Source: CAD feature listing. Evaluate the final solid. Frame: model axes, mm. Face numbers are marked on the shaded views. A direction names the side the tool comes from. Give positions to 0.01 mm unless a question says otherwise; leave off trailing zeros. Order: outer loops, then holes, each group sorted by start corner. A loop starts at its lowest first (then second) coordinate and runs counter-clockwise, first axis right, second up. Notation, with made-up numbers: (-8.75, 53) -> (5.25, 53) arc R16 cw to (5.25, 58) -> close; hole circle Ø6 at (8, -22). An arc over 180 degrees is marked (long way). Answer in a Markdown table with one row per item.
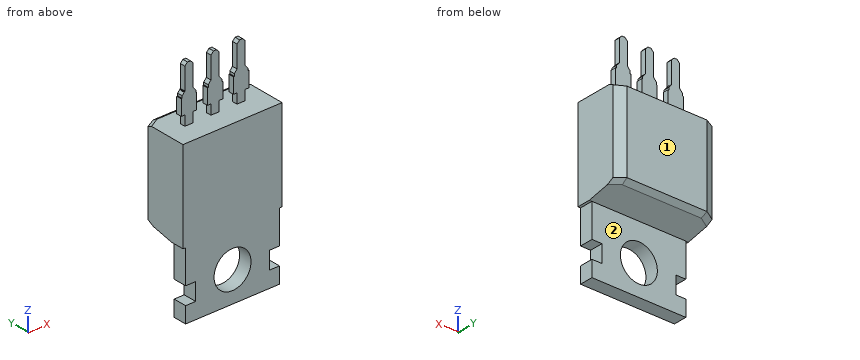
```python
from build123d import *
from OCP.BRepFilletAPI import BRepFilletAPI_MakeChamfer

# Parameters (mm, degrees)
EXTRUDE1_DEPTH      = 4.826
EXTRUDE1_DEPTH_BACK = 4.826
SKETCH10_R          = 1.8
SKETCH10_W          = 1.233836604
SKETCH10_H          = 1.6931216
EXTRUDE5_DEPTH      = 16.428369203
SKETCH6_W           = 0.8
SKETCH6_H           = 0.52
EXTRUDE6_DEPTH      = 5.38
EXTRUDE7_START      = -0.52
EXTRUDE7_DEPTH      = 0.52
CHAMFER1_SIZE       = 0.254
SKETCH12_W          = 7.379682426
SKETCH12_H          = 2.736118788
EXTRUDE8_DEPTH      = 0.254
SKETCH13_W          = 7.379682426
SKETCH13_H          = 2.736118788
EXTRUDE9_DEPTH      = 0.254
CHAMFER2_SIZE       = 0.508
CHAMFER2_SIZE2      = 0.91645626
CHAMFER3_SIZE       = 0.2032
CHAMFER3_SIZE2      = 0.366582504
CHAMFER3_SIZE2_2    = 0.605677555
CHAMFER3_SIZE2_3    = 0.557834937
EXTRUDE10_DEPTH     = 1.016


with BuildPart() as part:
    # Sketch2 → Extrude1 (new, two sides: drawn at the far end of the back side and taken through both)
    with BuildSketch(Plane(origin=(0, 0, 0), x_dir=(0, 0, -1), z_dir=(1, 0, 0)).offset(-EXTRUDE1_DEPTH_BACK)):
        Polygon((14.3005, 0), (-1.0795, 0), (-1.0795, 4.5), (7.124012877, 4.5), (7.8005, 1.3), (14.3005, 1.3), align=None)
    extrude(amount=EXTRUDE1_DEPTH + EXTRUDE1_DEPTH_BACK)

    # Sketch10 → Extrude5 (cut, through all)
    with BuildSketch(Plane(origin=(0, 1.3, 0), x_dir=(1, 0, 0), z_dir=(0, 1, 0))):
        with Locations(Location((0, 11.3505, 0), (0, 0, 270))):
            Circle(SKETCH10_R)
        with Locations((-4.209081698, 11.892729701)):
            Rectangle(SKETCH10_W, SKETCH10_H)
        with Locations((4.209081698, 11.892729701)):
            Rectangle(SKETCH10_W, SKETCH10_H)
    extrude(amount=-EXTRUDE5_DEPTH, mode=Mode.SUBTRACT)

    # Sketch6 → Extrude6 (add)
    with BuildSketch(Plane.XY.offset(1.0795)):
        with Locations((2.54, 2.25)):
            Rectangle(SKETCH6_W, SKETCH6_H)
        with Locations((-2.54, 2.25)):
            Rectangle(SKETCH6_W, SKETCH6_H)
        with Locations((0, 2.25)):
            Rectangle(SKETCH6_W, SKETCH6_H)
    extrude(amount=EXTRUDE6_DEPTH)

    # Sketch11 → Extrude7 (add)
    with BuildSketch(Plane(origin=(0, 2.51, 0), x_dir=(1, 0, 0), z_dir=(0, 1, 0)).offset(EXTRUDE7_START)):
        Polygon((-2.94, -2.0475), (-3.29, -2.0475), (-3.29, -3.5395), (-3.2004, -3.5395), (-3.2004, -3.7747), (-2.94, -4.0795), align=None)
        Polygon((-1.79, -2.0475), (-2.14, -2.0475), (-2.14, -4.0795), (-1.8796, -3.7747), (-1.8796, -3.5395), (-1.79, -3.5395), align=None)
        Polygon((-0.4, -2.0475), (-0.75, -2.0475), (-0.75, -3.5395), (-0.6604, -3.5395), (-0.6604, -3.7747), (-0.4, -4.0795), align=None)
        Polygon((0.75, -2.0475), (0.4, -2.0475), (0.4, -4.0795), (0.6604, -3.7747), (0.6604, -3.5395), (0.75, -3.5395), align=None)
        Polygon((2.14, -2.0475), (1.79, -2.0475), (1.79, -3.5395), (1.8796, -3.5395), (1.8796, -3.7747), (2.14, -4.0795), align=None)
        Polygon((3.29, -2.0475), (2.94, -2.0475), (2.94, -4.0795), (3.2004, -3.7747), (3.2004, -3.5395), (3.29, -3.5395), align=None)
    extrude(amount=EXTRUDE7_DEPTH)

    # Chamfer1
    chamfer1_edges = [part.edges().sort_by_distance(p)[0] for p in [
        (-2.14, 2.25, 6.4595),
        (-2.94, 2.25, 6.4595),
        (2.94, 2.25, 6.4595),
        (2.14, 2.25, 6.4595),
        (0.4, 2.25, 6.4595),
        (-0.4, 2.25, 6.4595),
    ]]
    chamfer(chamfer1_edges, length=CHAMFER1_SIZE)

    # Sketch12 → Extrude8 (cut)
    with BuildSketch(Plane.ZY.offset(4.826)):
        with Locations((-11.490341213, 1.368059394)):
            Rectangle(SKETCH12_W, SKETCH12_H)
    extrude(amount=-EXTRUDE8_DEPTH, mode=Mode.SUBTRACT)

    # Sketch13 → Extrude9 (cut)
    with BuildSketch(Plane(origin=(4.826, 0, 0), x_dir=(0, 0, -1), z_dir=(1, 0, 0))):
        with Locations((11.490341213, 1.368059394)):
            Rectangle(SKETCH13_W, SKETCH13_H)
    extrude(amount=-EXTRUDE9_DEPTH, mode=Mode.SUBTRACT)

    # Chamfer2: one chamfer whose edges measure the first distance from different faces: ONE call of the kernel's chamfer builder (chamfer() names one face for all edges)
    chamfer2_edges_1 = [part.edges().sort_by_distance(p)[0] for p in [
        (-4.826, 4.5, -3.022256439),
    ]]
    chamfer2_side_1 = [part.faces().sort_by_distance(p)[0] for p in [
        (-4.826, 2.217055195, -3.243165334),
    ]]
    chamfer2_edges_2 = [part.edges().sort_by_distance(p)[0] for p in [
        (4.826, 4.5, -3.022256439),
    ]]
    chamfer2_side_2 = [part.faces().sort_by_distance(p)[0] for p in [
        (4.826, 2.217055195, -3.243165334),
    ]]
    chamfer2 = BRepFilletAPI_MakeChamfer(part.part.solid().wrapped)
    for e in chamfer2_edges_1:
        chamfer2.Add(CHAMFER2_SIZE, CHAMFER2_SIZE2, e.wrapped, chamfer2_side_1[0].wrapped)  # the first distance lies on this face
    for e in chamfer2_edges_2:
        chamfer2.Add(CHAMFER2_SIZE, CHAMFER2_SIZE2, e.wrapped, chamfer2_side_2[0].wrapped)  # the first distance lies on this face
    add(Compound.cast(chamfer2.Shape()), mode=Mode.REPLACE)

    # Chamfer3: one chamfer whose edges measure the first distance from different faces: ONE call of the kernel's chamfer builder (chamfer() names one face for all edges)
    chamfer3_edges_1 = [part.edges().sort_by_distance(p)[0] for p in [
        (0, 4.5, 1.0795),
    ]]
    chamfer3_side_1 = [part.faces().sort_by_distance(p)[0] for p in [
        (0, 4.5, -3.022256439),
    ]]
    chamfer3_edges_2 = [part.edges().sort_by_distance(p)[0] for p in [
        (-4.36777187, 4.246, 1.0795),
    ]]
    chamfer3_side_2 = [part.faces().sort_by_distance(p)[0] for p in [
        (-4.368765147, 4.245449417, -3.049162718),
    ]]
    chamfer3_edges_3 = [part.edges().sort_by_distance(p)[0] for p in [
        (4.36777187, 4.246, 1.0795),
    ]]
    chamfer3_side_3 = [part.faces().sort_by_distance(p)[0] for p in [
        (4.368765147, 4.245449417, -3.049162718),
    ]]
    chamfer3_edges_4 = [part.edges().sort_by_distance(p)[0] for p in [
        (0, 4.5, -7.124012877),
    ]]
    chamfer3_side_4 = [part.faces().sort_by_distance(p)[0] for p in [
        (0, 4.5, -3.022256439),
    ]]
    chamfer3_edges_5 = [part.edges().sort_by_distance(p)[0] for p in [
        (-4.36777187, 4.246, -7.177709043),
    ]]
    chamfer3_side_5 = [part.faces().sort_by_distance(p)[0] for p in [
        (-4.368765147, 4.245449417, -3.049162718),
    ]]
    chamfer3_edges_6 = [part.edges().sort_by_distance(p)[0] for p in [
        (4.36777187, 4.246, -7.177709043),
    ]]
    chamfer3_side_6 = [part.faces().sort_by_distance(p)[0] for p in [
        (4.368765147, 4.245449417, -3.049162718),
    ]]
    chamfer3 = BRepFilletAPI_MakeChamfer(part.part.solid().wrapped)
    for e in chamfer3_edges_1:
        chamfer3.Add(CHAMFER3_SIZE, CHAMFER3_SIZE2, e.wrapped, chamfer3_side_1[0].wrapped)  # the first distance lies on this face
    for e in chamfer3_edges_2:
        chamfer3.Add(CHAMFER3_SIZE, CHAMFER3_SIZE2, e.wrapped, chamfer3_side_2[0].wrapped)  # the first distance lies on this face
    for e in chamfer3_edges_3:
        chamfer3.Add(CHAMFER3_SIZE, CHAMFER3_SIZE2, e.wrapped, chamfer3_side_3[0].wrapped)  # the first distance lies on this face
    for e in chamfer3_edges_4:
        chamfer3.Add(CHAMFER3_SIZE, CHAMFER3_SIZE2_2, e.wrapped, chamfer3_side_4[0].wrapped)  # the first distance lies on this face
    for e in chamfer3_edges_5:
        chamfer3.Add(CHAMFER3_SIZE, CHAMFER3_SIZE2_3, e.wrapped, chamfer3_side_5[0].wrapped)  # the first distance lies on this face
    for e in chamfer3_edges_6:
        chamfer3.Add(CHAMFER3_SIZE, CHAMFER3_SIZE2_3, e.wrapped, chamfer3_side_6[0].wrapped)  # the first distance lies on this face
    add(Compound.cast(chamfer3.Shape()), mode=Mode.REPLACE)

    # Sketch15 → Extrude10 (add)
    with BuildSketch(Plane.XY.offset(4.0795)):
        with BuildLine():
            Line((-2.14, 2.51), (-2.94, 2.51))
            ThreePointArc((-2.94, 2.51), (-3.017074418, 2.25), (-2.94, 1.99))
            Line((-2.94, 1.99), (-2.14, 1.99))
            ThreePointArc((-2.14, 1.99), (-2.062925582, 2.25), (-2.14, 2.51))
        make_face()
    extrude(amount=-EXTRUDE10_DEPTH)


solid = part.part
```
(1) Section query C-C (z = -10.75). Return the cut outline in (x, y), plus the area to 3 significant figures.
A:
| item | result |
|---|---|
| outline | (-4.57, 0) -> (-1.7, 0) -> (-1.7, 1.3) -> (-4.57, 1.3) -> close; (1.7, 0) -> (4.57, 0) -> (4.57, 1.3) -> (1.7, 1.3) -> close |
| area | 7.48 mm^2 |
(2) Section query A-A (z = 2.25). Return the cut outline in (x, y).
A:
| item | result |
|---|---|
| outline | (-3.29, 1.99) -> (-1.79, 1.99) -> (-1.79, 2.51) -> (-3.29, 2.51) -> close; (-0.75, 1.99) -> (0.75, 1.99) -> (0.75, 2.51) -> (-0.75, 2.51) -> close; (1.79, 1.99) -> (3.29, 1.99) -> (3.29, 2.51) -> (1.79, 2.51) -> close |
(3) Ray query, probe 1 along X at (y, z) = (2.05, 5); probe 2 along Y at (x, z) = (-4, -11); probe 3 along Y at (x, z) = (3.25, 3). Return the intervals inside material, ascending.
A:
| item | result |
|---|---|
| probe 1 | x = -2.94 to -2.14, -0.4 to 0.4, 2.14 to 2.94 |
| probe 2 | y = 0 to 1.3 |
| probe 3 | y = 1.99 to 2.51 |
(4) Section query B-B (y = 0.4). Return the cut outline in (x, z), plus the area to 3 significant figures.
A:
| item | result |
|---|---|
| outline | (-4.83, -7.8) -> (-4.57, -7.8) -> (-4.57, -11.05) -> (-3.59, -11.05) -> (-3.59, -12.74) -> (-4.57, -12.74) -> (-4.57, -14.3) -> (4.57, -14.3) -> (4.57, -12.74) -> (3.59, -12.74) -> (3.59, -11.05) -> (4.57, -11.05) -> (4.57, -7.8) -> (4.83, -7.8) -> (4.83, 1.08) -> (-4.83, 1.08) -> close; hole circle Ø3.6 at (0, -11.35) |
| area | 132 mm^2 |
(5) Access query for the marked faces 1 and 2. Directions: +Z, -Z, +X, -X, +Y, -Y. A direction counts if a zero-diameter tool reaches every point of the face in a straight line with its end or side. Return the directions, or none.
A:
| item | result |
|---|---|
| face 1 | +Z, -Z, +X, -X, +Y |
| face 2 | -Z, +X, -X, +Y |
(6) Section query D-D (y = 3.1). Return the cut outline in (x, z).
A:
| item | result |
|---|---|
| outline | (-4.83, -7.42) -> (4.83, -7.42) -> (4.83, 1.08) -> (-4.83, 1.08) -> close |
(7) First-contact query: pin 1 Ø1.4 at (y, z) = (0.5, -12) entering from -X; pin 2 Ø1.6 at (x, z) = (0, 4.5) entering from -Y; pin 3 Ø4 at (x, z) = (1.5, -11.5) entering from +Y; pin 4 Ø1.5 at (y, z) = (3.5, -9) entering from +X. Flat tips, straight axial feed; report the tip coordinate or a pass-through.
A:
| item | result |
|---|---|
| pin 1 | stops at x = -3.59 |
| pin 2 | stops at y = 1.99 |
| pin 3 | stops at y = 1.3 |
| pin 4 | passes through |
